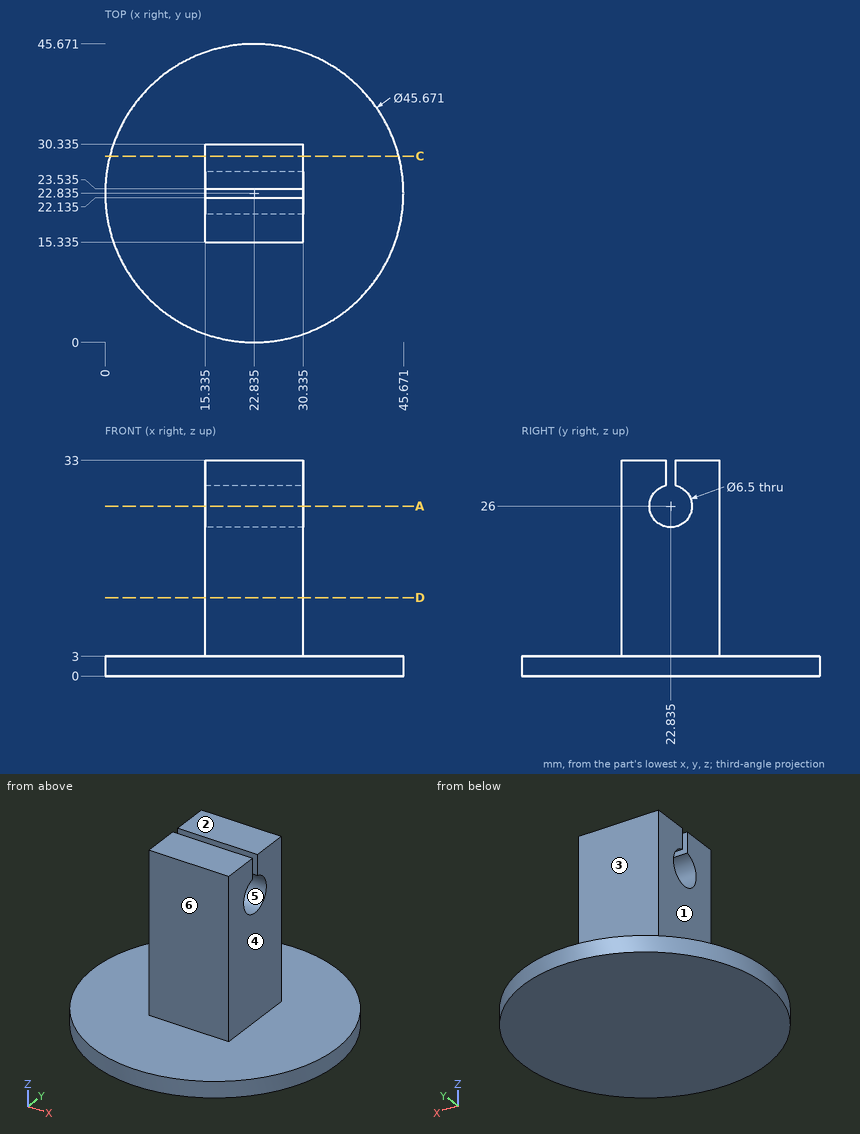
Can you work these out from the drawing? Everything is in mm from the part's minimum corner. A direction names the side the tool comes from. Give positions to 0.01 mm unless a question says otherwise; leave off trailing zeros. Order: outer loops, then holes, each group sorted by start corner. A loop starts at its lowest first (then second) coordinate and runs counter-clockwise, first axis right, second up. Notation, with made-up numbers: M -36.5,28 L 14.5,28 A19 ccw 14.5,48 Z; hole C -32,79.5 d7. An arc over 180 degrees is marked long. Write item = value, one per line. Start each with the question number.
Q1. Suppose I cut it at D-D (z = 12). Write out the boundary of the cut face in (x, y) (1 decimal), plus the area to 3 significant figures.
Q2. We'd pull the mould along Y, two halves only. Please class the marked faces 4, 5 and 6: pulls with the +Y half, pulls with the -Y half, needs draft (parallel to the pull), parting line crosses it, or undercut.
Q3. I need wall thicknesses on probe 1 along Y at (x, z) = (25, 26) (1 decimal); probe 2 along Z at (x, y) = (13, 24); probe 3 along X at (y, z) = (20, 5.5) (1 decimal). Which ranges of each line are inside material? Lowest first, please. Write a range as [from, to].
Q4. Suppose I cut it at C-C (y = 28.5). Write out the boundary of the cut face in (x, z) (1 decimal).
Q5. Will these pins go through, and if not, where does the flat tip stop? pin 1 Ø12 at (x, z) = (26, 11.5) entering from +Y (1 decimal); pin 2 Ø10 at (x, z) = (15, 6.5) entering from +Y; pin 3 Ø10.5 at (y, z) = (22.84, 26) entering from +X (1 decimal); pin 4 Ø6 at (x, z) = (11, 17) entering from -Y.
Q6. For the marked faces 1, 2 and 3, which set-ups out of +Z, -Z, +X, -X, +Y, -Y let a thin tool reach every point of the face, with its end or its side?
Q7. Suppose I cut it at A-A (z = 26). Write out the boundary of the cut face in (x, y) (1 decimal).
Check result:
q1.outline = M 15.3,15.3 L 30.3,15.3 L 30.3,30.3 L 15.3,30.3 Z
q1.area = 225 mm2
q2.face_4 = needs draft
q2.face_5 = undercut
q2.face_6 = pulls with the -Y half
q3.probe_1 = [15.3, 19.6], [26.1, 30.3]
q3.probe_2 = [0, 3]
q3.probe_3 = [15.3, 30.3]
q4.outline = M 0.7,0 L 45,0 L 45,3 L 30.3,3 L 30.3,33 L 15.3,33 L 15.3,3 L 0.7,3 Z
q5.pin_1 = 30.3
q5.pin_2 = 45.27
q5.pin_3 = 30.3
q5.pin_4 = through
q6.face_1 = +Z, -X, +Y, -Y
q6.face_2 = +Z, +X, -X, +Y, -Y
q6.face_3 = +Z, +X, -X, +Y
q7.outline = M 15.3,15.3 L 30.3,15.3 L 30.3,19.6 L 15.3,19.6 Z; M 15.3,26.1 L 30.3,26.1 L 30.3,30.3 L 15.3,30.3 Z
